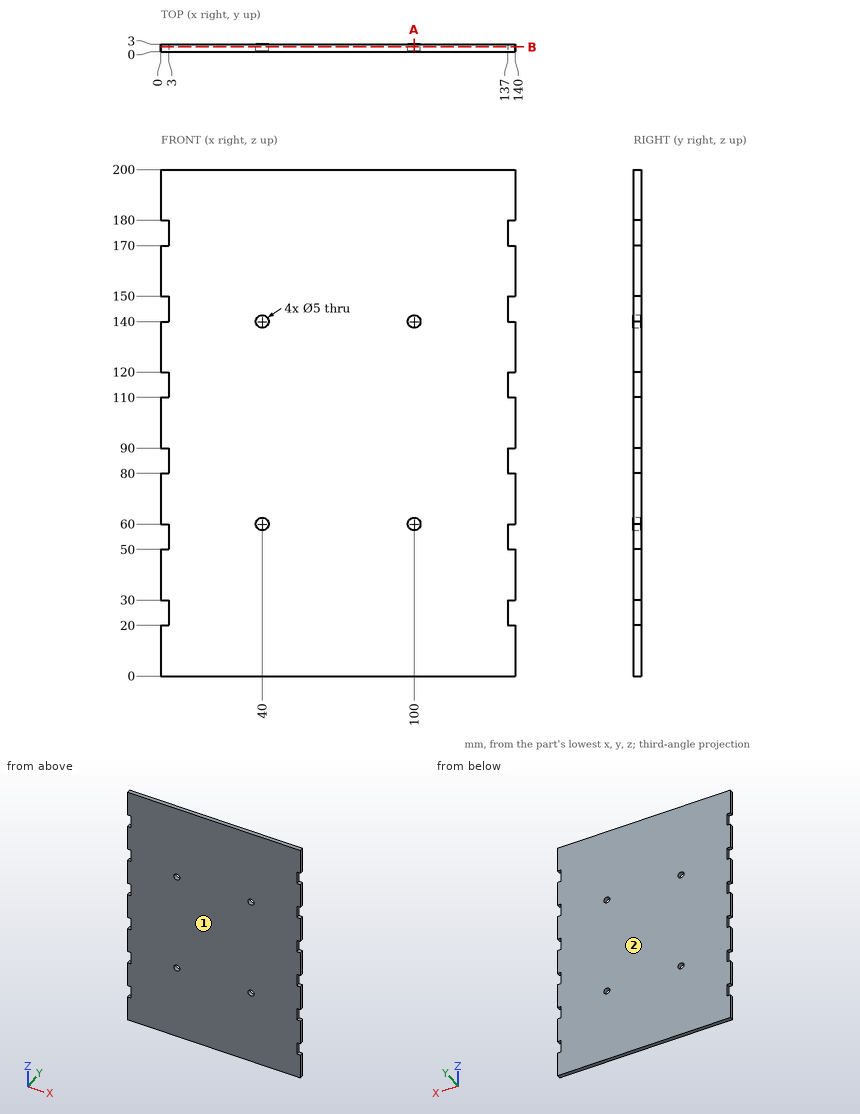
Input: dimensioned drawing with shaded views. Units: mm. Origin: part minimum x, y, z. Coordinates: 2 decimals unless noted, no trailing zeros. Loops run counter-clockwise (first coordinate to the right, second up) from the corner with the lowest first, then second, coordinate; pieces in that order, holes last. Notation, with made-up numbers: (68.25, 4.5) -> (91.25, 4.5) arc R36 ccw to (91.25, 40.5) -> close; hole circle Ø8 at (85.5, 7.5). An arc over 180 degrees is marked (long way). Use a Markdown table: item, result. Add a question column.
(1) Line query: line 1 along X through (y, z) = (1.6, 171); line 2 along Z through (x, y) = (98.5, 1.85); line 3 along Z through (x, y) = (40.5, 2.05). Output: solid intervals per line, ascending.
(2) Section query A-A, the plane x = 100. Return loops of the section in (y, z).
(3) Pin query (flat end, axial travel): pin 1 Ø0.9 at (x, y) = (139, 2) entering from -Z; pin 2 Ø1.5 at (y, z) = (2, 117) entering from -X. Return the tip coordinate at first contact, or that it passes through.
(4) Section query B-B, the plane y = 1.85. State how many separate pieces and enclosed holes the cut face has, plus the area to 3 significant figures.
(5) Mould query, pull axis Y, two halves, no side actions, for the marked faces 1 and 2. Classes: pulls with the +Y half, pulls with the -Y half, needs draft (parallel to the pull), parting line crosses it, or undercut.
Answer:
| question | item | result |
|---|---|---|
| 1 | line 1 | x = 3 to 137 |
| 1 | line 2 | z = 0 to 58, 62 to 138, 142 to 200 |
| 1 | line 3 | z = 0 to 57.55, 62.45 to 137.55, 142.45 to 200 |
| 2 | outline | (0, 0) -> (3, 0) -> (3, 57.5) -> (0, 57.5) -> close; (0, 62.5) -> (3, 62.5) -> (3, 137.5) -> (0, 137.5) -> close; (0, 142.5) -> (3, 142.5) -> (3, 200) -> (0, 200) -> close |
| 3 | pin 1 | stops at z = 0 |
| 3 | pin 2 | stops at x = 3 |
| 4 | separate pieces | 1 |
| 4 | enclosed holes | 4 |
| 4 | area | 27,600 mm^2 |
| 5 | face 1 | pulls with the -Y half |
| 5 | face 2 | pulls with the +Y half |
